from build123d import *

# Parameters (mm, degrees)
IZIM1_W                       = 19
IZIM1_H                       = 3.8
Y_KSEKLIK_EKSTR_ZYON1_DEPTH   = 50
Y_KSEKLIK_EKSTR_ZYON1_2_DEPTH = 50
Y_KSEKLIK_EKSTR_ZYON2_DEPTH   = 3
IZIM3_R                       = 6.5
KES_EKSTR_ZYON1_DEPTH         = 5
IZIM4_R                       = 4
KES_EKSTR_ZYON2_DEPTH         = 5
IZIM5_W                       = 19
IZIM5_H                       = 6
KES_EKSTR_ZYON3_DEPTH         = 73
IZIM6_W                       = 19
IZIM6_H                       = 7
KES_EKSTR_ZYON4_DEPTH         = 9
Y_KSEKLIK_EKSTR_ZYON3_DEPTH   = 19


with BuildPart() as part:
    # izim1 → Y_kseklik-Ekstr_zyon1 (new body)
    with BuildSketch(Plane(origin=(0, 0, 0), x_dir=(1, 0, 0), z_dir=(0, 1, 0))):
        with Locations((0, 58.9)):
            Rectangle(IZIM1_W, IZIM1_H)
    extrude(amount=Y_KSEKLIK_EKSTR_ZYON1_DEPTH)



with BuildPart() as body_2:
    # izim1 → Y_kseklik-Ekstr_zyon1 2 (new body)
    with BuildSketch(Plane(origin=(0, 0, 0), x_dir=(1, 0, 0), z_dir=(0, 1, 0))):
        with Locations((0, -1.9)):
            Rectangle(IZIM1_W, IZIM1_H)
    extrude(amount=Y_KSEKLIK_EKSTR_ZYON1_2_DEPTH)


with BuildPart() as part_1:
    add(part.part)

    add(body_2.part)  # Y_kseklik-Ekstr_zyon2 merges body 2
    # izim2 → Y_kseklik-Ekstr_zyon2 (add)
    with BuildSketch(Plane(origin=(0, 50, 0), x_dir=(1, 0, 0), z_dir=(0, 1, 0))):
        Polygon((-9.5, 60.8), (-9.5, 41), (-12.5, 41), (-12.5, 16), (-9.5, 16), (-9.5, -3.8), (9.5, -3.8), (9.5, 16), (12.5, 16), (12.5, 41), (9.5, 41), (9.5, 60.8), align=None)
    extrude(amount=Y_KSEKLIK_EKSTR_ZYON2_DEPTH)

    # izim3 → Kes-Ekstr_zyon1 (cut)
    with BuildSketch(Plane(origin=(0, 0, -60.8), x_dir=(-1, 0, 0), z_dir=(0, 0, -1))):
        with Locations((0, 25)):
            Circle(IZIM3_R)
    extrude(amount=-KES_EKSTR_ZYON1_DEPTH, mode=Mode.SUBTRACT)

    # izim4 → Kes-Ekstr_zyon2 (cut)
    with BuildSketch(Plane(origin=(0, 0, 0), x_dir=(-1, 0, 0), z_dir=(0, 0, -1))):
        with Locations((0, 25)):
            Circle(IZIM4_R)
    extrude(amount=-KES_EKSTR_ZYON2_DEPTH, mode=Mode.SUBTRACT)

    # izim5 → Kes-Ekstr_zyon3 (cut)
    with BuildSketch(Plane(origin=(0, 0, -60.8), x_dir=(-1, 0, 0), z_dir=(0, 0, -1))):
        with Locations((0, 3)):
            Rectangle(IZIM5_W, IZIM5_H)
    extrude(amount=-KES_EKSTR_ZYON3_DEPTH, mode=Mode.SUBTRACT)

    # izim6 → Kes-Ekstr_zyon4 (cut)
    with BuildSketch(Plane.XY.offset(3.8)):
        with Locations((0, 9.5)):
            Rectangle(IZIM6_W, IZIM6_H)
    extrude(amount=-KES_EKSTR_ZYON4_DEPTH, mode=Mode.SUBTRACT)

    # izim7 → Y_kseklik-Ekstr_zyon3 (add)
    with BuildSketch(Plane(origin=(9.5, 0, 0), x_dir=(0, 0, -1), z_dir=(1, 0, 0))):
        Polygon((57, 50), (57, 43), (50, 50), align=None)
        Polygon((0, 50), (0, 43), (7, 50), align=None)
    extrude(amount=-Y_KSEKLIK_EKSTR_ZYON3_DEPTH)


solid = part_1.part
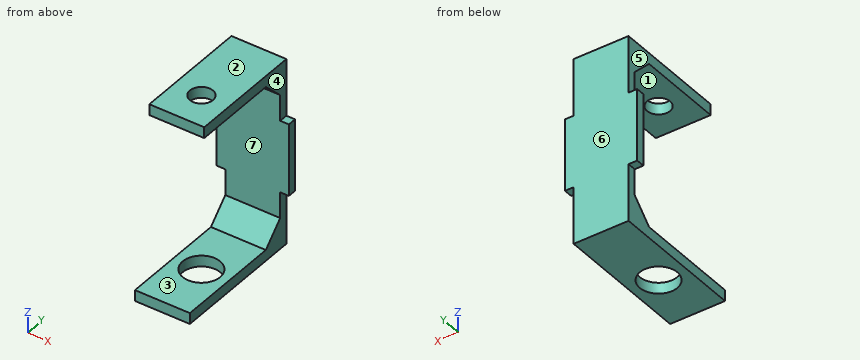
The listing builds one solid part. Answer for the finished solid, in the listing's coordinates (mm). Face numbers are marked on the shaded views. A direction names the side the tool comes from. Round coordinates to 2 decimals unless told otherwise and drop trailing zeros. Order: outer loops, then holes, each group sorted by start corner. A loop starts at its lowest first (then second) coordinate and runs counter-clockwise, first axis right, second up. Notation, with made-up numbers: M 80.5,60 L 105.5,60 A23 ccw 105.5,71 Z; hole C 17,-13.5 d11. An arc over 180 degrees is marked long. Answer in a Markdown table with one row per item. Add a question column.
1) The part is cut by section C-C on y = 25. Determine the outline of the cut face in (x, z).
2) Which of the six approach directions +Z, -Z, +X, -X, +Y, -Y give full straight-line access (tool end or side, diameter ignored) to the marked faces 5, 6 and 7?
3) Determine the mould class of the marked faces 1, 2, 3 and 4 for opening direction Z: pulls with the +Z half, pulls with the -Z half, needs draft (parallel to the pull), parting line crosses it, or undercut.
4) Flat-ended cylindrical pins translate along their axes: pin 1 Ø11.5 at (x, y) = (0, 25) entering from -Z; pin 2 Ø3 at (x, z) = (-2.5, -54) entering from -Y; pin 3 Ø2.5 at (x, y) = (11.5, 52) entering from +Z. Find the tip coordinate at first contact, or state that the pin passes through.
5) Consider line 1 along Z through (x, y) = (-3.5, 33); line 2 along Y through (x, z) = (0, 1.55); line 3 along Y through (x, z) = (0.75, -45.5). Determine where each line is inside the solid, lowest interval first. Write a range as from..to.
6) The part is cut by section A-A on y = 45.5. Determine the outline of the cut face in (x, z), plus the area to 3 significant figures.
7) The part is cut by section B-B on x = 0. Determine the outline of the cut face in (y, z), plus the area to 3 significant figures.
8) The part is cut by section D-D on x = 5.5. Determine the outline of the cut face in (y, z), plus the area to 3 significant figures.
Findings below:
| question | item | result |
|---|---|---|
| 1 | outline | M -9.5,-60.8 L -6.5,-60.8 L -6.5,-57 L -9.5,-57 Z; M -9.5,0 L -4,0 L -4,3.8 L -9.5,3.8 Z; M 4,0 L 9.5,0 L 9.5,3.8 L 4,3.8 Z; M 6.5,-60.8 L 9.5,-60.8 L 9.5,-57 L 6.5,-57 Z |
| 2 | face 5 | +Z, -X, +Y, -Y |
| 2 | face 6 | +Z, -Z, +X, -X, +Y |
| 2 | face 7 | +X, -X, -Y |
| 3 | face 1 | undercut |
| 3 | face 2 | pulls with the +Z half |
| 3 | face 3 | undercut |
| 3 | face 4 | needs draft |
| 4 | pin 1 | stops at z = 0 |
| 4 | pin 2 | stops at y = 44.5 |
| 4 | pin 3 | stops at z = -16 |
| 5 | line 1 | z = -60.8..-57, 0..3.8 |
| 5 | line 2 | y = 13..21, 29..53 |
| 5 | line 3 | y = 50..53 |
| 6 | outline | M -9.5,-60.8 L 9.5,-60.8 L 9.5,-54.5 L -9.5,-54.5 Z; M -9.5,-2.5 L 9.5,-2.5 L 9.5,3.8 L -9.5,3.8 Z |
| 6 | area | 239 mm² |
| 7 | outline | M 6,-60.8 L 18.5,-60.8 L 18.5,-57 L 6,-57 Z; M 13,0 L 21,0 L 21,3.8 L 13,3.8 Z; M 29,0 L 43,0 L 50,-7 L 50,-50 L 43,-57 L 31.5,-57 L 31.5,-60.8 L 53,-60.8 L 53,3.8 L 29,3.8 Z |
| 7 | area | 471 mm² |
| 8 | outline | M 6,-60.8 L 21.54,-60.8 L 21.54,-57 L 6,-57 Z; M 13,0 L 43,0 L 50,-7 L 50,-50 L 43,-57 L 28.46,-57 L 28.46,-60.8 L 53,-60.8 L 53,3.8 L 13,3.8 Z |
| 8 | area | 524 mm² |
